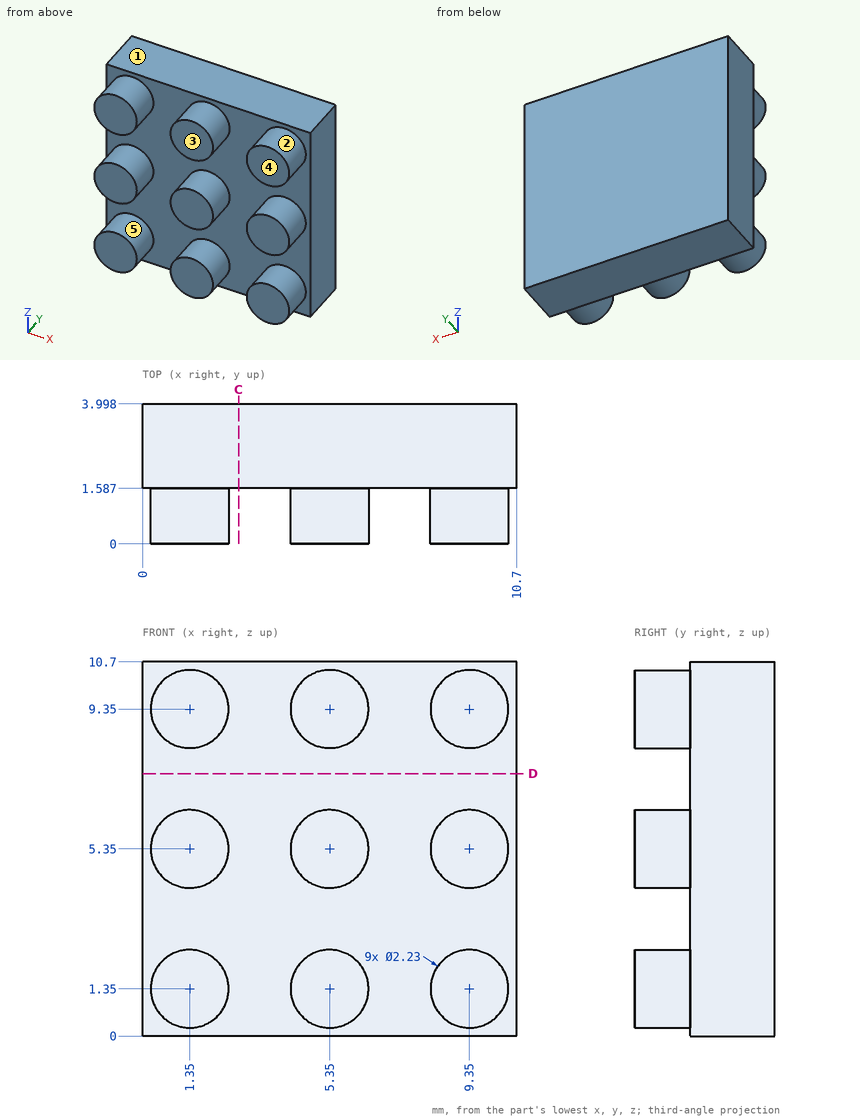
The figure shows three views and two pictorial views of one solid part (mm, origin at its lowest corner). Answer the questions. A direction names the side the tool comes from. Coordinates: 2 decimals unless noted, no trailing zeros. Loops run counter-clockwise (first coordinate to the right, second up) from the corner with the lowest first, then second, coordinate; pieces in that order, holes last.
(1) The mould has two halves that part along Z. Classify the marked faces 1, 2 and 3: released by +Z, released by -Z, zero draft, split by the parting line, or undercut.
Solution:
face 1: released by +Z
face 2: undercut
face 3: zero draft
(2) Consider line 1 along Z through (x, y) = (9.5, 0.6) (1 decimal); line 2 along Z through (x, y) = (9.75, 1.15); line 3 along Y through (x, z) = (3, 3). Determine where each line is inside the solid, lowest interval first.
Solution:
line 1: z = 0.2 to 2.5, 4.2 to 6.5, 8.2 to 10.5
line 2: z = 0.31 to 2.39, 4.31 to 6.39, 8.31 to 10.39
line 3: y = 1.59 to 4
(3) A tool of negligible diameter and unlimited length cuts with its end or side. For the marked faces 4 and 5, from which of +Z, -Z, +X, -X, +Y, -Y can it reach the whole face along a straight path? Write none if from no direction.
Solution:
face 4: +Z, -Z, +X, -X, -Y
face 5: -Y
(4) The part is cut by section C-C (x = 2.75). Determine the outline of the cut face in (y, z).
Solution:
outline: (1.59, 0) - (4, 0) - (4, 10.7) - (1.59, 10.7) - close
(5) The part is cut by section D-D (z = 7.5). Determine the outline of the cut face in (x, y).
Solution:
outline: (0, 1.59) - (10.7, 1.59) - (10.7, 4) - (0, 4) - close
(6) A flat-ended cylindrical pin translates along its axis: pin 1 Ø1.5 at (x, y) = (3, 0.5) entering from +Z. Find the tip coordinate at first contact, or state that the pin passes through.
Solution:
pin 1: stops at z = 10.01
